Source: CAD feature listing. Evaluate the final solid. Frame: model axes, mm. A direction names the side the tool comes from. Round coordinates to 2 decimals unless told otherwise and drop trailing zeros. Loops run counter-clockwise (first coordinate to the right, second up) from the corner with the lowest first, then second, coordinate; pieces in that order, holes last. Notation, with made-up numbers: (8, -2.5) -> (65, -2.5) arc R17 cw to (65, 14.5) -> close; hole circle Ø2 at (15, 24). An arc over 180 degrees is marked (long way). Return JSON: item names as keys, results as strings. Group by question number.
```python
from build123d import *

# Parameters (mm, degrees)
F0_W     = 25.4
F0_H     = 31.75
F0_R     = 10.5
F1_DEPTH = 7.62
F3_D     = 4.7625
F3_DEPTH = 4.7625
F3_TIP   = 1.4307993491
F0_R_2   = 9
F4_DEPTH = 1.27


# Not quite as in the source:
# - a feature names something its author has since deleted; it is built from what else it names


with BuildPart() as f1:
    # F0 (on Right) → F1 (new body)
    with BuildSketch(Plane.YZ):
        Rectangle(F0_W, F0_H)
        Circle(F0_R, mode=Mode.SUBTRACT)
    extrude(amount=F1_DEPTH)

    # F3
    with Locations(Plane(origin=(0, 0, -15.875), x_dir=(1, 0, 0), z_dir=(0, 0, -1))):
        with Locations((3.81, 6.35), (3.81, -6.35)):
            Hole(F3_D / 2, depth=F3_DEPTH)
            with Locations((0, 0, -(F3_DEPTH + F3_TIP / 2))):  # 118° drill point
                Cone(0, F3_D / 2, F3_TIP, mode=Mode.SUBTRACT)

    # F0 (on Right) → F4 (join)
    with BuildSketch(Plane.YZ):
        Circle(F0_R)
        Circle(F0_R_2, mode=Mode.SUBTRACT)
    extrude(amount=F4_DEPTH)


solid = f1.part
```
(1) Cut plane A-A (y = 0). Return loops of the section in (x, z) (3 decimals).
(2) Ray query, line 1 (Y direction, x = 3.81, z = -12.5); line 2 (Z direction, x = 0.75, y = 0) (3 decimals); line 3 (X direction, y = -9.25, z = 0.5). Return the intervals inside material, ascending.
(3) Cut plane B-B (z = 6). Return loops of the section in (x, y), and give its area (3 significant figures).
(4) Pin query (flat end, axial travel): pin 1 (4 mm diameter, centred on x = 3.81, y = -6.35, fed in from -Z); pin 2 (10.5 mm diameter, centred on y = 1.5, z = 4.5, fed in from +X); pin 3 (11 mm diameter, centred on y = 0, z = 0, fed in from +X). Return the tip coordinate at first contact, or that it passes through.
(5) Set-up query: faces 1 (the face through (1.27, 8, 5)), 2 (the face through (1.54, 5.63, -13.46)), 3 (the face through (4, -12.7, 0)). Return all of +Z, -Z, +X, -X, +Y, -Y with unobstructed straight access to the full face (end or side cutting, diameter ignored); none if empty.
(6) Cut plane C-C (x = 7). Return loops of the section in (y, z) (3 decimals), and give its area (3 significant figures).
(7) Mould query, pull axis Y, two halves, no side actions, for faces 4 (the face through (4, 0, -15.875)), 5 (the face through (4.4, 10, 3.2)), 6 (the face through (1.61, -5.44, -13.46)), 7 (the face through (4, 12.7, 0)). Classes: released by +Y, released by -Y, zero draft, split by the parting line, or undercut.
Answers follow:
{
 "1": {"outline": "(0, -15.875) -> (7.62, -15.875) -> (7.62, -10.5) -> (1.27, -10.5) -> (1.27, -9) -> (0, -9) -> close; (0, 9) -> (1.27, 9) -> (1.27, 10.5) -> (7.62, 10.5) -> (7.62, 15.875) -> (0, 15.875) -> close"},
 "2": {"line 1": "-12.7 to -8.73, -3.97 to 3.97, 8.73 to 12.7", "line 2": "-15.875 to -9, 9 to 15.875", "line 3": "0 to 1.27"},
 "3": {"outline": "(0, -12.7) -> (7.62, -12.7) -> (7.62, -8.62) -> (1.27, -8.62) -> (1.27, -6.71) -> (0, -6.71) -> close; (0, 6.71) -> (1.27, 6.71) -> (1.27, 8.62) -> (7.62, 8.62) -> (7.62, 12.7) -> (0, 12.7) -> close", "area": "67.1 mm^2"},
 "4": {"pin 1": "z = -10.88", "pin 2": "x = 1.27", "pin 3": "through"},
 "5": {"face 1": "+X", "face 2": "-Z", "face 3": "+Z, -Z, +X, -X, -Y"},
 "6": {"outline": "(-12.7, -15.875) -> (12.7, -15.875) -> (12.7, 15.875) -> (-12.7, 15.875) -> close; hole circle Ø21 at (0, 0)", "area": "460 mm^2"},
 "7": {"face 4": "zero draft", "face 5": "undercut", "face 6": "undercut", "face 7": "released by +Y"}
}
